Autodesk Inventor part; units mm, degrees
ref_plane "YZ Plane" through (0, 0, 0) normal (1, 0, 0) x (0, 1, 0)
ref_plane "XZ Plane" through (0, 0, 0) normal (0, 1, 0) x (-1, 0, 0)
ref_plane "XY Plane" through (0, 0, 0) normal (0, 0, 1) x (1, 0, 0)
sketch "Sketch1" plane through (0, 0, 0) normal (0, 0, 1) x (1, 0, 0)
  line L0 (0, 0) -> (-41.402, 0)
  line L1 (-41.402, 0) -> (-177.8, 93.599)
  line L2 (-177.8, 93.599) -> (-177.8, 135.001)
  line L3 (-177.8, 135.001) -> (0, 135.001)
  line L4 (0, 135.001) -> (0, 0)
  circle A0 centre (-20.701, 12.7) radius 3.3655
  circle A1 centre (-20.701, 63.5) radius 3.3655
  circle A2 centre (-20.701, 114.3) radius 3.3655
  circle A3 centre (-71.501, 114.3) radius 3.3655
  circle A4 centre (-122.301, 114.3) radius 3.3655
  circle A5 centre (-173.101, 114.3) radius 3.3655
  dimension "d0" = 41.402
  dimension "d1" = 41.402
  dimension "d2" = 177.8
  dimension "d3" = 135.001
  dimension "d4" = 6.731
  dimension "d6" = 20.701
  dimension "d9" = 50.8
  dimension "d14" = 20.701
  dimension "d15" = 20.701
  dimension "d16" = 50.8
  dimension "d17" = 12.7
  dimension "d20" = 50.8
  dimension "d25" = 4.699
extrude "Extrusion1" add sketch "Sketch1" along normal blind 2.286
fillet "Fillet1" radius 3.175 5 edges at (0, 135.001, 1.143) (0, 0, 1.143) (-41.402, 0, 1.143) (-177.8, 93.599, 1.143) (-177.8, 135.001, 1.143)
sketch "Sketch2" plane through (0, 0, 2.286) normal (0, 0, 1) x (1, 0, 0)
  circle A0 centre (-122.301, 114.3) radius 3.3655 construction
  circle A1 centre (-122.301, 114.3) radius 4.953
  point P0 (0, 0)
  dimension "d29" = 1.5875
extrude "Extrusion2" cut sketch "Sketch2" against normal through all
properties part number "Corner-Tower-Brace Upper" material "Aluminum 6061"
Build history of the part. All positions in model axes, mm. Round coordinates to 2 decimals unless told otherwise and drop trailing zeros. Loops run counter-clockwise (first coordinate to the right, second up) from the corner with the lowest first, then second, coordinate; pieces in that order, holes last. Notation, with made-up numbers: (76, 57.5) -> (111, 57.5) arc R9 ccw to (111, 73.5) -> close; hole circle Ø10 at (44.25, -3). An arc over 180 degrees is marked (long way). One line per item, written item: value. Start each with the question number.
Q1. Drop a flat-ended pin along its axis: pin 1 Ø6 at (x, y) = (-20.701, 63.5) entering from -Z. Give the stop position or say it passes through.
Q2. Cut at A-A on z = 0.5. Count the separate pieces of the cut face and the enclosed holes in it, plus the area to 3 significant figures.
Q3. Probe line 1 along Y through (x, z) = (-126.5, 1.2); line 2 along X through (y, z) = (61, 1.2); line 3 along X through (y, z) = (65.5, 0.2). List the from-to ranges inside material, lowest first.
Q4. Cut at C-C on x = -121. List the corners of the cut face in (y, z), plus the area to 3 significant figures.
Q5. Cut at B-B on y = 114.3. List the corners of the cut face in (x, z), plus the area to 3 significant figures.
Q6. Two-plate mould, pull along Y, no slides. Class faces 1 (the face through (-108.38, 45.96, 1.13)), 2 (the face through (-70, 83, 0)), 3 (the face through (-18.892, 9.862, 1.127)), 4 (the face through (-117.577, 115.788, 1.159)): released by +Y, released by -Y, zero draft, split by the parting line, or undercut.
Q7. Cut at D-D on y = 63.5. List the corners of the cut face in (x, z).
Computed:
1. pin 1: through
2. separate pieces: 1
2. enclosed holes: 6
2. area: 17,400 mm²
3. line 1: 58.4 to 111.67, 116.93 to 135
3. line 2: -130.29 to -22.95, -18.45 to 0
3. line 3: -136.85 to -23.41, -17.99 to 0
4. outline: (54.62, 0) -> (109.52, 0) -> (109.52, 2.29) -> (54.62, 2.29) -> close; (119.08, 0) -> (135, 0) -> (135, 2.29) -> (119.08, 2.29) -> close
4. area: 162 mm²
5. outline: (-177.8, 0) -> (-176.47, 0) -> (-176.47, 2.29) -> (-177.8, 2.29) -> close; (-169.74, 0) -> (-127.25, 0) -> (-127.25, 2.29) -> (-169.74, 2.29) -> close; (-117.35, 0) -> (-74.87, 0) -> (-74.87, 2.29) -> (-117.35, 2.29) -> close; (-68.14, 0) -> (-24.07, 0) -> (-24.07, 2.29) -> (-68.14, 2.29) -> close; (-17.34, 0) -> (0, 0) -> (0, 2.29) -> (-17.34, 2.29) -> close
5. area: 338 mm²
6. face 1: released by -Y
6. face 2: zero draft
6. face 3: undercut
6. face 4: undercut
7. outline: (-133.94, 0) -> (-24.07, 0) -> (-24.07, 2.29) -> (-133.94, 2.29) -> close; (-17.34, 0) -> (0, 0) -> (0, 2.29) -> (-17.34, 2.29) -> close
